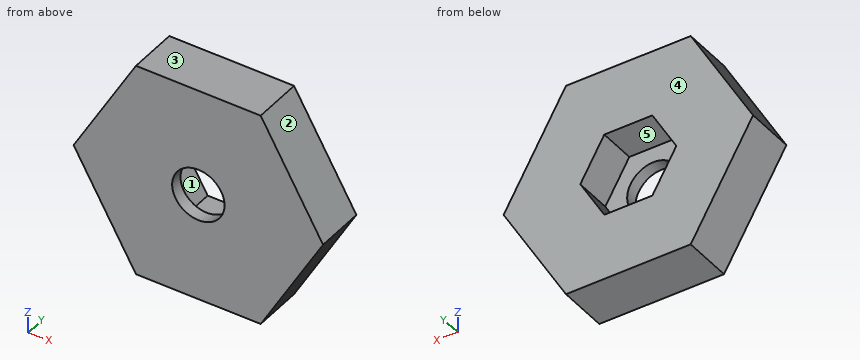
```python
from build123d import *

# Parameters (mm, degrees)
BOSS_EXTRUDE1_DEPTH = 6
SKETCH2_R           = 4.2
BOSS_EXTRUDE2_DEPTH = 2


with BuildPart() as part:
    # Sketch1 → Boss-Extrude1 (new body)
    with BuildSketch(Plane(origin=(0, 0, 0), x_dir=(1, 0, 0), z_dir=(0, 1, 0))):
        Polygon((-10, 17.320508076), (-20, 0), (-10, -17.320508076), (10, -17.320508076), (20, 0), (10, 17.320508076), align=None)
        Polygon((-3.85, 6.668395609), (-7.7, 0), (-3.85, -6.668395609), (3.85, -6.668395609), (7.7, 0), (3.85, 6.668395609), align=None, mode=Mode.SUBTRACT)
    extrude(amount=BOSS_EXTRUDE1_DEPTH)

    # Sketch2 → Boss-Extrude2 (add)
    with BuildSketch(Plane.XZ):
        Polygon((20, 0), (10, -17.320508076), (-10, -17.320508076), (-20, 0), (-10, 17.320508076), (10, 17.320508076), align=None)
        Circle(SKETCH2_R, mode=Mode.SUBTRACT)
    extrude(amount=BOSS_EXTRUDE2_DEPTH)


solid = part.part
```
Can you work these out from the model? Positions are in its coordinate system, mm. Face numbers are marked on the shaded views. A direction names the side the tool comes from. Give positions to 0.01 mm unless a question says otherwise; leave off trailing zeros. Loops run counter-clockwise (first coordinate to the right, second up) from the corner with the lowest first, then second, coordinate; pieces in that order, holes last. Notation, with made-up numbers: M 34.25,68 L 89.25,68 A16 ccw 89.25,72 Z; hole C 8.25,9 d11. An arc over 180 degrees is marked long. One line per item, written item: value.
(1) We'd pull the mould along Z, two halves only. Please class the marked faces 3, 4 and 5: released by +Z, released by -Z, zero draft, split by the parting line, or undercut.
Returned:
face 3: released by +Z
face 4: zero draft
face 5: undercut
(2) Will these pins go through, and if not, where does the flat tip stop? pin 1 (4 mm diameter, centred on x = 15.5, y = 1.5, fed in from -Z); pin 2 (3 mm diameter, centred on x = 10.5, y = 1, fed in from -Z); pin 3 (3 mm diameter, centred on y = 1.5, z = -8, fed in from -X).
Returned:
pin 1: z = -11.26
pin 2: z = -17.32
pin 3: x = -16.25
(3) Suppose I cut it at D-D on x = -6. List the corners of the cut face in (y, z) for me, plus the area to 3 significant figures.
Returned:
outline: M -2,-17.32 L 6,-17.32 L 6,-2.94 L 0,-2.94 L 0,2.94 L 6,2.94 L 6,17.32 L -2,17.32 Z
area: 242 mm^2
(4) I need wall thicknesses on line 1 (Z direction, x = 0, y = -1); line 2 (Z direction, x = -2, y = 2.5); line 3 (X direction, y = 3.5, z = -2). Which ranges of each line are inside material? Lowest first, please.
Returned:
line 1: -17.32 to -4.2, 4.2 to 17.32
line 2: -17.32 to -6.67, 6.67 to 17.32
line 3: -18.85 to -6.55, 6.55 to 18.85
(5) Suppose I cut it at A-A on x = 0. List the corners of the cut face in (y, z) for me, plus the area to 3 significant figures.
Returned:
outline: M -2,-17.32 L 6,-17.32 L 6,-6.67 L 0,-6.67 L 0,-4.2 L -2,-4.2 Z; M -2,4.2 L 0,4.2 L 0,6.67 L 6,6.67 L 6,17.32 L -2,17.32 Z
area: 180 mm^2
(6) Suppose I cut it at C-C on y = 2.25. List the corners of the cut face in (x, z) for me, plus the area to 3 significant figures.
Returned:
outline: M -20,0 L -10,-17.32 L 10,-17.32 L 20,0 L 10,17.32 L -10,17.32 Z; hole M -7.7,0 L -3.85,-6.67 L 3.85,-6.67 L 7.7,0 L 3.85,6.67 L -3.85,6.67 Z
area: 885 mm^2
(7) Suppose I cut it at B-B on y = -1. List the corners of the cut face in (x, z) for me, plus the area to 3 significant figures.
Returned:
outline: M -20,0 L -10,-17.32 L 10,-17.32 L 20,0 L 10,17.32 L -10,17.32 Z; hole C 0,0 d8.4
area: 984 mm^2
(8) Which directions (+Z, -Z, +X, -X, +Y, -Y) give clear straight access to the entire face, cutting with the end or side of a thin tool? Please do the marked faces 1 and 2.
Returned:
face 1: +Y
face 2: +Z, +X, +Y, -Y
